Input: part model. Units: mm. Frame: model coordinates. A direction names the side the tool comes from. Round coordinates to 2 decimals unless told otherwise and drop trailing zeros. Loops run counter-clockwise (first coordinate to the right, second up) from the corner with the lowest first, then second, coordinate; pieces in that order, holes last. Notation, with made-up numbers: (48.25, -36.5) - (104.25, -36.5) arc R16 cw to (104.25, -17.5) - close; hole circle Ø6 at (74, 18.5). An arc over 180 degrees is marked (long way). Write each question's results on one line, items separated by ' | '.
from build123d import *

# Parameters (mm, degrees)
CHAMFER1_SIZE = 1.524


with BuildPart() as part:
    # Sketch1 → Revolve1 (revolve)
    with BuildSketch(Plane.XY):
        with BuildLine():
            Line((0, 0), (12.7, 0))
            Line((12.7, 0), (12.7, -4.572))
            Line((12.7, -4.572), (19.05, -4.572))
            Line((19.05, -4.572), (19.05, 0))
            Line((19.05, 0), (38.1, 0))
            ThreePointArc((38.1, 0), (35.758167108, 2.772791168), (32.280128867, 3.81))
            Line((32.280128867, 3.81), (0, 3.81))
            Line((0, 3.81), (0, 0))
        make_face()
    revolve(axis=Axis((-29.818959813, -12.7, 0), (1, 0, 0)))

    # Chamfer1
    chamfer1_edges = [part.edges().sort_by_distance(p)[0] for p in [
        (0, -25.4, 0),
    ]]
    chamfer(chamfer1_edges, length=CHAMFER1_SIZE)


solid = part.part
1. Set-up query: faces 5 (the cylindrical face through (15.92, -5.19, -3.11)), 6 (the flat face through (19.05, -21, 0)). Return all of +Z, -Z, +X, -X, +Y, -Y with unobstructed straight access to the full face (end or side cutting, diameter ignored); none if empty.
Answer:
face 5: +X, -X | face 6: +X
2. Section query B-B, the plane y = -12.7. Output: boundary loops of the cut face in (x, z), plus the area to 3 significant figures.
Answer:
outline: (0, -16.51) - (32.28, -16.51) arc R6.35 ccw to (38.1, -12.7) - (19.05, -12.7) - (19.05, -8.13) - (12.7, -8.13) - (12.7, -12.7) - (1.52, -12.7) - (0, -14.22) - close; (0, 14.22) - (1.52, 12.7) - (12.7, 12.7) - (12.7, 8.13) - (19.05, 8.13) - (19.05, 12.7) - (38.1, 12.7) arc R6.35 ccw to (32.28, 16.51) - (0, 16.51) - close | area: 334 mm^2
3. Mould query, pull axis Z, two halves, no side actions, for faces 1 (the flat face through (12.7, -4, 0)), 2 (the flat face through (0, -8, 14)), 3 (the cylindrical face through (15.914, 3.048, 4.959)), 4 (the cylindrical face through (7.19, -0.586, 3.815)). Classes: pulls with the +Z half, pulls with the -Z half, needs draft (parallel to the pull), parting line crosses it, or undercut.
Answer:
face 1: undercut | face 2: needs draft | face 3: parting line crosses it | face 4: undercut
4. Section query C-C, the plane x = 4. Output: boundary loops of the cut face in (y, z).
Answer:
outline: circle Ø33.02 at (-12.7, 0); hole circle Ø25.4 at (-12.7, 0)
5. Line query: line 1 (X direction, y = -21, z = -9.5); line 2 (Z direction, x = 7.75, y = -12.7); line 3 (Y direction, x = 27.5, z = -2). Output: solid intervals per line, ascending. Write a range as [from, to].
Answer:
line 1: [12.7, 19.05] | line 2: [-16.51, -12.7], [12.7, 16.51] | line 3: [-29.09, -25.24], [-0.16, 3.69]
6. Section query A-A, the plane z = 0. Output: boundary loops of the cut face in (x, y), plus the area to 3 significant figures.
Answer:
outline: (0, -29.21) - (32.28, -29.21) arc R6.35 ccw to (38.1, -25.4) - (19.05, -25.4) - (19.05, -20.83) - (12.7, -20.83) - (12.7, -25.4) - (1.52, -25.4) - (0, -26.92) - close; (0, 1.52) - (1.52, 0) - (12.7, 0) - (12.7, -4.57) - (19.05, -4.57) - (19.05, 0) - (38.1, 0) arc R6.35 ccw to (32.28, 3.81) - (0, 3.81) - close | area: 334 mm^2
7. Contact query for flat-ended pins moving along their axis: pin 1 (1 mm diameter, centred on y = -7.5, z = 2.5, fed in from +X); pin 2 (12.5 mm diameter, centred on y = -6.5, z = -2.5, fed in from +X); pin 3 (12 mm diameter, centred on x = 27, z = -7.5, fed in from -Y); pin 4 (6 mm diameter, centred on x = 12.5, y = -18, fed in from +Z). Output: stop coordinate, or through.
Answer:
pin 1: through | pin 2: x = 38.1 | pin 3: y = -29.14 | pin 4: z = 16.35
